```python
from build123d import *

# Parameters (mm, degrees)
F0_W     = 321.573243
F0_H     = 239.584401
F1_DEPTH = 2.5
F2_W     = 30
F2_H     = 90
F3_DEPTH = 30
F4_W     = 30
F4_H     = 90
F5_DEPTH = 30
F6_R     = 4.370205
F6_R_2   = 4.469907
F6_R_3   = 3.832918
F6_R_4   = 2.234953
F6_R_5   = 4.678676
F6_R_6   = 4.678688
F7_DEPTH = 30


with BuildPart() as f1:
    # F0 (on Top) → F1 (new body)
    with BuildSketch(Plane.XY):
        with Locations((-9.229324, -49.054674)):
            Rectangle(F0_W, F0_H)
    extrude(amount=F1_DEPTH)

    # F2 (on face) → F3 (cut)
    with BuildSketch(Plane.XY.offset(2.5)):
        with Locations((-131.251947, -15.25378)):
            Rectangle(F2_W, F2_H)
    extrude(amount=-F3_DEPTH, mode=Mode.SUBTRACT)

    # F4 (on Top) → F5 (cut)
    with BuildSketch(Plane.XY):
        with Locations((114.714116, -16.105251)):
            Rectangle(F4_W, F4_H)
    extrude(amount=F5_DEPTH, mode=Mode.SUBTRACT)

    # F6 (on face) → F7 (cut)
    with BuildSketch(Plane.XY.offset(2.5)):
        with Locations((-163.504452, 62.698148)):
            Circle(F6_R)
        with Locations((140.44629, 63.464731)):
            Circle(F6_R_2)
        with Locations((-8.654387, 65.381192)):
            Circle(F6_R_3)
        with Locations((-7.504508, -161.144525)):
            Circle(F6_R_4)
        with Locations((-163.504452, -160.377949)):
            Circle(F6_R_5)
        with Locations((140.829593, -160.377949)):
            Circle(F6_R_6)
    extrude(amount=-F7_DEPTH, mode=Mode.SUBTRACT)


solid = f1.part
```
CAD build for the part. Positions are in the model's coordinates, mm. Coordinates: 2 decimals unless noted, no trailing zeros. Order: outer loops, then holes, each group sorted by start corner. A loop starts at its lowest first (then second) coordinate and runs counter-clockwise, first axis right, second up. Notation, with made-up numbers: (84, 40) - (121, 40) arc R28 ccw to (121, 60) - close; hole circle Ø6 at (3, 63). An arc over 180 degrees is marked (long way). Use a Markdown table: item, result. Add a question column.
(1) Saw through at C-C (z = 2.1). Count the separate pieces of the cut face and the enclosed holes in it, then the cut area to 3 significant figures.
(2) Saw through at A-A (x = -141). Give the cut face in (y, z).
(3) Saw through at B-B (y = -42.5). Give the cut face in (x, z).
(4) Drill centre lines: line 1 along X through (y, z) = (-29.5, 1.45); line 2 along Y through (x, z) = (107, 0.95); line 3 along Y through (x, z) = (137, 0.85). Where is each one in solid material? Low to high. Write a range as [from, to].
(5) Pull direction Y, two halves, no side cores. Call faces 1 (the face through (-11, -47, 2.5)), 2 (the face through (-161.35, -164.53, 1.27)): +Y half, -Y half, draft (parallel to the pull), parting line (faces both ways), or undercut.
Solved:
| question | item | result |
|---|---|---|
| 1 | separate pieces | 1 |
| 1 | enclosed holes | 8 |
| 1 | area | 71,300 mm² |
| 2 | outline | (-168.85, 0) - (-60.25, 0) - (-60.25, 2.5) - (-168.85, 2.5) - close; (29.75, 0) - (70.74, 0) - (70.74, 2.5) - (29.75, 2.5) - close |
| 3 | outline | (-170.02, 0) - (-146.25, 0) - (-146.25, 2.5) - (-170.02, 2.5) - close; (-116.25, 0) - (99.71, 0) - (99.71, 2.5) - (-116.25, 2.5) - close; (129.71, 0) - (151.56, 0) - (151.56, 2.5) - (129.71, 2.5) - close |
| 4 | line 1 | x = [-170.02, -146.25], [-116.25, 99.71], [129.71, 151.56] |
| 4 | line 2 | y = [-168.85, -61.11], [28.89, 70.74] |
| 4 | line 3 | y = [-168.85, -163.07], [-157.69, 60.62], [66.31, 70.74] |
| 5 | face 1 | draft |
| 5 | face 2 | undercut |
